from build123d import *

# Parameters (mm, degrees)
BOSS_EXTRUDE1_DEPTH = 2.5
FILLET1_R           = 1


with BuildPart() as part:
    # Sketch1 → Revolve1 (revolve)
    with BuildSketch(Plane.XY, mode=Mode.PRIVATE) as revolve1_sk:
        with BuildLine():
            Line((0, 0), (5, 0))
            ThreePointArc((5, 0), (8.535533906, 1.464466094), (10, 5))
            Line((10, 5), (10, 33.285700302))
            ThreePointArc((10, 33.285700302), (5.625709026, 36.973401218), (3.989031047, 42.455631126))
            Line((3.989031047, 42.455631126), (3.989031047, 207))
            Line((3.989031047, 207), (6, 207))
            Line((6, 207), (6, 209))
            Line((6, 209), (0, 209))
            Line((0, 209), (0, 0))
        make_face()
    revolve(revolve1_sk.sketch.rotate(Axis((0, 0, 0), (0, -1, 0)), 90), axis=Axis((0, 0, 0), (0, -1, 0)))

    # Sketch2 → Boss-Extrude1 (add, symmetric)
    with BuildSketch(Plane.XY):
        with BuildLine():
            Line((-6, 209), (6, 209))
            ThreePointArc((6, 209), (0, 212), (-6, 209))
        make_face()
    extrude(amount=BOSS_EXTRUDE1_DEPTH, both=True)

    # Fillet1
    # the kernel refuses this fillet: 1 mm, written as the material it takes off along each edge
    with BuildSketch(Plane(origin=(0, 204.5, -2.5), x_dir=(0.9523393361832132, 0.3050406346015508, 0), z_dir=(0.3050406346015508, -0.9523393361832132, 0))) as fillet1_piece_1_section:
        with BuildLine():
            CenterArc((7.5 - FILLET1_R, FILLET1_R), FILLET1_R, 270, 90)
            Line((7.5 - FILLET1_R, 0), (7.5, 0))
            Line((7.5, 0), (7.5, FILLET1_R))
        make_face()
    fillet1_piece_1 = revolve(axis=Axis((0, 204.5, -2.5), (0, 0, 1)), revolution_arc=144.478782805, mode=Mode.PRIVATE)
    fillet1_piece_1 = split(fillet1_piece_1, bisect_by=Plane(origin=(5.716310171, 209, -2.240967586), z_dir=(0, 1, 0)), keep=Keep.TOP, mode=Mode.PRIVATE)
    add(fillet1_piece_1, mode=Mode.SUBTRACT)
    with BuildSketch(Plane(origin=(0, 204.5, 2.5), x_dir=(0.9523393361832132, 0.3050406346015508, 0), z_dir=(0.3050406346015508, -0.9523393361832132, 0))) as fillet1_piece_2_section:
        with BuildLine():
            CenterArc((7.5 - FILLET1_R, -FILLET1_R), FILLET1_R, 0, 90)
            Line((7.5, -FILLET1_R), (7.5, 0))
            Line((7.5, 0), (7.5 - FILLET1_R, 0))
        make_face()
    fillet1_piece_2 = revolve(axis=Axis((0, 204.5, 2.5), (0, 0, 1)), revolution_arc=144.478782805, mode=Mode.PRIVATE)
    fillet1_piece_2 = split(fillet1_piece_2, bisect_by=Plane(origin=(5.71631017, 209, 2.240967722), z_dir=(0, 1, 0)), keep=Keep.TOP, mode=Mode.PRIVATE)
    add(fillet1_piece_2, mode=Mode.SUBTRACT)


solid = part.part
Geometry: final body of the model. Coordinates: model frame, mm. Give positions to 0.01 mm unless a question says otherwise; leave off trailing zeros. Order: outer loops, then holes, each group sorted by start corner. A loop starts at its lowest first (then second) coordinate and runs counter-clockwise, first axis right, second up. Notation, with made-up numbers: (69.25, 61) -> (75.25, 61) arc R16 ccw to (75.25, 90) -> close; hole circle Ø5 at (20, 33.25). An arc over 180 degrees is marked (long way). Write each question's results on one line, items separated by ' | '.
1) Line query: line 1 along Z through (x, y) = (0.5, 142); line 2 along Y through (x, z) = (-1, 5.25); line 3 along Z through (x, y) = (-5.25, 22.5). Output: solid intervals per line, ascending.
Geometry says:
line 1: z = -3.96 to 3.96 | line 2: y = 0.01 to 37.43, 207 to 209 | line 3: z = -8.51 to 8.51
2) Cut plane C-C (y = 24). Output: boundary loops of the cut face in (x, z).
Geometry says:
outline: circle Ø20 at (0, 0)
3) Draft query along Y for faces 1 (the face through (3.9, 207, 1.4)), 2 (the face through (0, 0, 0)), 3 (the face through (0, 209, 4)), 4 (the face through (0, 19, -10)). Return one class per face: released by +Y, released by -Y, zero draft, split by the parting line, or undercut.
Geometry says:
face 1: undercut | face 2: released by -Y | face 3: released by +Y | face 4: zero draft
4) Cut plane A-A (x = 0). Output: boundary loops of the cut face in (y, z).
Geometry says:
outline: (0, -5) arc R5 ccw to (5, -10) -> (33.29, -10) arc R10 cw to (42.46, -3.99) -> (207, -3.99) -> (207, -6) -> (209, -6) -> (209, -2.5) -> (211, -2.5) arc R1 ccw to (212, -1.5) -> (212, 1.5) arc R1 ccw to (211, 2.5) -> (209, 2.5) -> (209, 6) -> (207, 6) -> (207, 3.99) -> (42.46, 3.99) arc R10 cw to (33.29, 10) -> (5, 10) arc R5 ccw to (0, 5) -> close
5) Cut plane B-B (y = 98). Output: boundary loops of the cut face in (x, z), and give its area (3 significant figures).
Geometry says:
outline: circle Ø7.98 at (0, 0) | area: 50.0 mm²
6) First-contact query: pin 1 Ø4 at (x, z) = (0.5, 7.5) entering from +Y; pin 2 Ø5 at (x, z) = (3, 4.5) entering from +Y; pin 3 Ø10 at (x, y) = (-3, 113) entering from +Z. Flat tips, straight axial feed; report the tip coordinate or a pass-through.
Geometry says:
pin 1: stops at y = 209 | pin 2: stops at y = 211.44 | pin 3: stops at z = 3.99
